Build history of the part. All positions in model axes, mm. Give positions to 0.01 mm unless a question says otherwise; leave off trailing zeros. Order: outer loops, then holes, each group sorted by start corner. A loop starts at its lowest first (then second) coordinate and runs counter-clockwise, first axis right, second up. Notation, with made-up numbers: M -13.75,51 L 45.25,51 A9 ccw 45.25,67 Z; hole C -9,20.5 d1. An arc over 180 degrees is marked long. One line per item, written item: value.
from build123d import *

# Parameters (mm, degrees)
SKETCH1_R      = 21.5
SKETCH1_R_2    = 13.75
EXTRUDE1_DEPTH = 6
EXTRUDE2_DEPTH = 31.991934435


with BuildPart() as part:
    # Sketch1 → Extrude1 (new body)
    with BuildSketch(Plane(origin=(0, 0, 0), x_dir=(1, 0, 0), z_dir=(0, 1, 0))):
        with Locations(Location((0, 0, 0), (0, 0, 270))):
            Circle(SKETCH1_R)
        with Locations(Location((0, 0, 0), (0, 0, 270))):
            Circle(SKETCH1_R_2, mode=Mode.SUBTRACT)
    extrude(amount=EXTRUDE1_DEPTH)

    # Sketch2 → Extrude2 (cut, through all)
    with BuildSketch(Plane(origin=(0, 0, 0), x_dir=(0, 0, -1), z_dir=(1, 0, 0))):
        Polygon((-8.196152423, 0), (-2.196152423, 0), (8.196152423, 6), (2.196152423, 6), align=None)
    extrude(amount=-EXTRUDE2_DEPTH, mode=Mode.SUBTRACT)


solid = part.part
1) Drill centre lines: probe 1 along Z at (x, y) = (0, 1.5); probe 2 along Z at (x, y) = (-5, 4); probe 3 along X at (y, z) = (3, 0). Where is each one in solid material? Low to high. Write a range as from..to.
Check values:
probe 1: -21.5..-13.75, 13.75..21.5
probe 2: -20.91..-12.81, 12.81..20.91
probe 3: 13.75..21.5
2) Saw through at A-A, the plane x = -14.5. Write the cut outline in (y, z).
Check values:
outline: M 0,-15.87 L 6,-15.87 L 6,-8.2 L 0,2.2 Z; M 0,8.2 L 6,-2.2 L 6,15.87 L 0,15.87 Z
3) Mould opens along Y. For faces 1 (the face through (-17, 3, -3)), 2 (the face through (0, 6, 14)), 3 (the face through (-17, 3, 3)), 4 (the face through (10, 0, -10)) say: released by +Y, released by -Y, zero draft, split by the parting line, or undercut.
Check values:
face 1: undercut
face 2: released by +Y
face 3: undercut
face 4: released by -Y
4) Saw through at B-B, the plane z = 11.5. Write the cut outline in (x, y), then the cut area to 3 significant figures.
Check values:
outline: M -18.17,0 L -7.54,0 L -7.54,6 L -18.17,6 Z; M 7.54,0 L 18.17,0 L 18.17,6 L 7.54,6 Z
area: 128 mm^2
5) Saw through at D-D, the plane y = 4.75. Write the cut outline in (x, z).
Check values:
outline: M -21.5,-0.03 L -13.75,-0.03 A13.75 cw long -12.36,-6.03 L -20.64,-6.03 A21.5 ccw long Z
6) Saw through at C-C, the plane z = 0. Write the cut outline in (x, y).
Check values:
outline: M -21.5,0 L -13.75,0 L -13.75,1.27 L -21.5,1.27 Z; M -21.5,4.73 L -13.75,4.73 L -13.75,6 L -21.5,6 Z; M 13.75,0 L 21.5,0 L 21.5,6 L 13.75,6 Z
7) Pin check, flat tips, straight feed: pin 1 (2 mm diameter, centred on y = 1, z = 1.5, fed in from +X); pin 2 (22 mm diameter, centred on x = 0, z = 0, fed in from +Y); pin 3 (1 mm diameter, centred on y = 2.5, z = 11, fed in from +X); pin 4 (2 mm diameter, centred on x = 5, z = 16, fed in from -Y). Stop position of each tip, or through.
Check values:
pin 1: x = 21.49
pin 2: through
pin 3: x = 18.76
pin 4: y = 0
